```python
from build123d import *

# Parameters (mm, degrees)
F1_DEPTH  = 50
F2_R      = 5
F2_R_2    = 1.45
F3_DEPTH  = 15
F2_R_3    = 10.05
F4_DEPTH  = 5
F5_R      = 11.05
F5_R_2    = 5
F6_DEPTH  = 2.3
F7_R      = 1.95
F8_DEPTH  = 34
F9_R      = 2.505
F10_DEPTH = 10
F11_R     = 1.45
F12_DEPTH = 22.958324159


with BuildPart() as f1:
    # F0 (on Right) → F1 (new body)
    with BuildSketch(Plane.YZ):
        Polygon((-15, 150), (-15, 10), (-155, 10), (-155, 0), (0, 0), (0, 150), align=None)
    extrude(amount=F1_DEPTH)

    # F2 (on face) → F3 (cut, through all)
    with BuildSketch(Plane.XZ.offset(15)):
        with Locations((25, 130)):
            Circle(F2_R)
        with Locations((9.5, 145.5)):
            Circle(F2_R_2)
        with Locations((9.5, 114.5)):
            Circle(F2_R_2)
        with Locations((40.5, 114.5)):
            Circle(F2_R_2)
        with Locations((40.5, 145.5)):
            Circle(F2_R_2)
    extrude(amount=-F3_DEPTH, mode=Mode.SUBTRACT)

    # F2 (on face) → F4 (cut)
    with BuildSketch(Plane.XZ.offset(15)):
        with Locations((25, 130)):
            Circle(F2_R_3)
        with Locations((25, 130)):
            Circle(F2_R, mode=Mode.SUBTRACT)
    extrude(amount=-F4_DEPTH, mode=Mode.SUBTRACT)

    # F5 (on face) → F6 (cut)
    with BuildSketch(Plane(origin=(0, 0, 0), x_dir=(-1, 0, 0), z_dir=(0, 1, 0))):
        with Locations((-25, 130)):
            Circle(F5_R)
        with Locations((-25, 130)):
            Circle(F5_R_2, mode=Mode.SUBTRACT)
    extrude(amount=-F6_DEPTH, mode=Mode.SUBTRACT)

    # F7 (on face) → F8 (cut)
    with BuildSketch(Plane.XZ.offset(155)):
        with Locations((12.5, 5)):
            Circle(F7_R)
        with Locations((37.5, 5)):
            Circle(F7_R)
    extrude(amount=-F8_DEPTH, mode=Mode.SUBTRACT)

    # F9 (on face) → F10 (cut, through all)
    with BuildSketch(Plane.XY.offset(10)):
        with Locations((25, -85)):
            Circle(F9_R)
    extrude(amount=-F10_DEPTH, mode=Mode.SUBTRACT)

    # F11 (on face) → F12 (cut, through all)
    with BuildSketch(Plane.YZ.offset(50)):
        with Locations((-85, 5)):
            Circle(F11_R)
    extrude(amount=-F12_DEPTH, mode=Mode.SUBTRACT)


solid = f1.part
```
Read the model definition and answer for the solid it produces. Units are mm, in the model's axes. A direction names the side the tool comes from. Coordinates: 2 decimals unless noted, no trailing zeros. Write each loop counter-clockwise with the first axis right and the second up, starting at its lowest first coordinate (ties: lowest second). Pieces come first, ordered by that corner, then holes. Notation, with made-up numbers: (48.5, 80.25) - (61.5, 80.25) arc R23 cw to (61.5, 97.25) - close; hole circle Ø10 at (49, -31.75). An arc over 180 degrees is marked (long way). Answer as a JSON object with one key per item and string values. Group by question number.
1. Each of these flat-tipped pins is pushed along its axis until it touches: P1, Ø8, axis at x = 16.5, y = -62, coming from the -Z side; P2, Ø22, axis at x = 26, z = 128.5, coming from the -Y side; P3, Ø16, axis at x = 25, z = 130, coming from the -Y side; P4, Ø17.5, axis at x = 25, z = 130, coming from the +Y side. Where does it stop, or does it pass through?
2. The mould has two halves that part along Z. Classify faces 1 (the cylindrical face through (39.3, -138.24, 4.25)), 2 (the cylindrical face through (19.901, -1.134, 120.197)), 3 (the flat face through (50, -14.7, 47.6)), 4 (the flat face through (25, -79, 0)): +Z half, -Z half, draft (parallel to the pull), parting line (faces both ways), or undercut.
3. A cutting plane is placed at A-A (x = 25). Determine the outline of the cut face in (y, z) (3 decimals).
4. Consider L1, parallel to Z at x = 40.5, y = -11; L2, parallel to Z at x = 12.5, y = -136; L3, parallel to Y at x = 26.5, z = 96. Determine where each line is inside the solid, lowest interval first. Write a range as [from, to].
5. Which of the six approach directions +Z, -Z, +X, -X, +Y, -Y give full straight-line access (tool end or side, diameter ignored) to faces 5 (the flat face through (20, -2.3, 128)), 6 (the cylindrical face through (22.82, -12.54, 120.19)), 7 (the flat face through (25, -15, 81))?
6. A cutting plane is placed at B-B (y = -133). Determine the outline of the cut face in (x, z).
7. A cutting plane is placed at C-C (y = -56). Determine the outline of the cut face in (x, z), plus the area to 3 significant figures.
8. A cutting plane is placed at D-D (z = 15). Determine the outline of the cut face in (x, y), plus the area to 3 significant figures.
Worked out:
{
 "1": {"P1": "stops at z = 0", "P2": "stops at y = -15", "P3": "stops at y = -10", "P4": "stops at y = -2.3"},
 "2": {"face 1": "undercut", "face 2": "undercut", "face 3": "draft", "face 4": "-Z half"},
 "3": {"outline": "(-155, 0) - (-87.505, 0) - (-87.505, 10) - (-155, 10) - close; (-82.495, 0) - (0, 0) - (0, 118.95) - (-2.3, 118.95) - (-2.3, 125) - (-10, 125) - (-10, 119.95) - (-15, 119.95) - (-15, 10) - (-82.495, 10) - close; (-15, 140.05) - (-10, 140.05) - (-10, 135) - (-2.3, 135) - (-2.3, 141.05) - (0, 141.05) - (0, 150) - (-15, 150) - close"},
 "4": {"L1": "z = [0, 113.05], [115.95, 144.05], [146.95, 150]", "L2": "z = [0, 3.05], [6.95, 10]", "L3": "y = [-15, 0]"},
 "5": {"face 5": "+Y", "face 6": "-Y", "face 7": "+Z, +X, -X, -Y"},
 "6": {"outline": "(0, 0) - (50, 0) - (50, 10) - (0, 10) - close; hole circle Ø3.9 at (12.5, 5); hole circle Ø3.9 at (37.5, 5)"},
 "7": {"outline": "(0, 0) - (50, 0) - (50, 10) - (0, 10) - close", "area": "500 mm²"},
 "8": {"outline": "(0, -15) - (50, -15) - (50, 0) - (0, 0) - close", "area": "750 mm²"}
}
